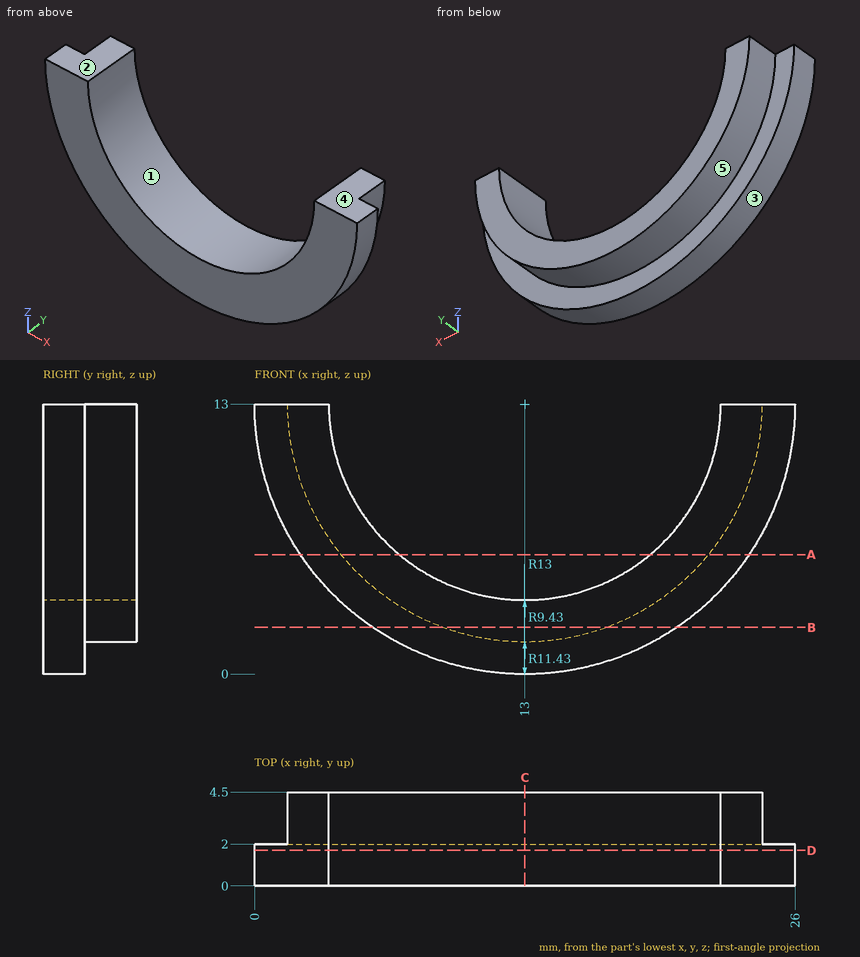
For this review, use the dimensioned drawing (mm, ordinates from the lowest corner) and the shaded views. A direction names the side the tool comes from. Give positions to 0.01 mm unless a question says otherwise; leave off trailing zeros. Write each loop counter-clockwise with the first axis right and the second up, starting at its lowest first coordinate (ties: lowest second). Pieces come first, ordered by that corner, then holes. Notation, with made-up numbers: M 64.25,62 L 120.25,62 A26 cw 120.25,88 Z; hole C -1.75,-38 d8. An arc over 180 degrees is marked long. Write item = value, one per line. Start each with the question number.
Q1. Machinability: for the marked faces 4 and 5, which of the approach directions +Z, -Z, +X, -X, +Y, -Y give a long, thin tool a straight path to every point of the face, cutting with its end or side? Answer none if there is none.
Q2. We need section B-B (z = 2.25). State the section outline as (x, y) points.
Q3. We need section D-D (y = 1.7). State the section outline as (x, z) points.
Q4. For line 1 (Z direction, x = 12.75, y = 2.7); line 2 (X direction, y = 4.15, z = 11.25); line 3 (X direction, y = 0.3, z = 12), list the stretches that pass through material, from the lowest coordinate up.
Q5. Mouldability with a two-part tool opening along X and no side actions: class the marked faces 1, 2 and 3 as released by +X, released by -X, zero draft, split by the parting line, or undercut.
Q6. We need section A-A (z = 5.75). State the section outline as (x, y) points, plus the area to 3 significant figures.
Q7. We need section C-C (x = 13). State the section outline as (y, z) points.
Result set:
q1.face_4 = +Z, +X, -X, +Y, -Y
q1.face_5 = -Z, +Y
q2.outline = M 5.69,0 L 20.31,0 L 20.31,2 L 16.88,2 L 16.88,4.5 L 9.12,4.5 L 9.12,2 L 5.69,2 Z
q3.outline = M 0,13 A13 ccw 26,13 L 22.43,13 A9.43 cw 3.57,13 Z
q4.line_1 = 1.57 to 3.57
q4.line_2 = 1.7 to 3.73, 22.27 to 24.3
q4.line_3 = 0.04 to 3.62, 22.38 to 25.96
q5.face_1 = undercut
q5.face_2 = zero draft
q5.face_3 = split by the parting line
q6.outline = M 2.21,0 L 6.97,0 L 6.97,4.5 L 4.16,4.5 L 4.16,2 L 2.21,2 Z; M 19.03,0 L 23.79,0 L 23.79,2 L 21.84,2 L 21.84,4.5 L 19.03,4.5 Z
q6.area = 33.1 mm2
q7.outline = M 0,0 L 2,0 L 2,1.57 L 4.5,1.57 L 4.5,3.57 L 0,3.57 Z
